from build123d import *

# Parameters (mm, degrees)
ESQUISSE1_R                       = 17
BOSS_EXTRU_1_DEPTH                = 17
ESQUISSE2_R                       = 12.5
BOSS_EXTRU_2_DEPTH                = 11.5
ESQUISSE3_R                       = 12
BOSS_EXTRU_3_DEPTH                = 3.5
ESQUISSE4_R                       = 12.5
BOSS_EXTRU_4_DEPTH                = 1.5
ESQUISSE5_R                       = 10.25
ENL_V_MAT_EXTRU_1_DEPTH           = 30
ESQUISSE6_R                       = 10.25
ESQUISSE6_R_2                     = 6.75
ENL_V_MAT_EXTRU_2_DEPTH           = 1.5
ESQUISSE7_R                       = 12
ESQUISSE7_R_2                     = 10.25
ENL_V_MAT_EXTRU_3_DEPTH           = 2
DIAM_TRE_DU_PER_AGE_3_0_3_1_D     = 3
DIAM_TRE_DU_PER_AGE_3_0_3_1_DEPTH = 12
DIAM_TRE_DU_PER_AGE_3_0_3_1_TIP   = 0.901290929


with BuildPart() as part:
    # Esquisse1 → Boss.-Extru.1 (new body)
    with BuildSketch(Plane.XY):
        Circle(ESQUISSE1_R)
    extrude(amount=BOSS_EXTRU_1_DEPTH)

    # Esquisse2 → Boss.-Extru.2 (add)
    with BuildSketch(Plane.XY.offset(17)):
        Circle(ESQUISSE2_R)
    extrude(amount=BOSS_EXTRU_2_DEPTH)

    # Esquisse3 → Boss.-Extru.3 (add)
    with BuildSketch(Plane.XY.offset(28.5)):
        Circle(ESQUISSE3_R)
    extrude(amount=BOSS_EXTRU_3_DEPTH)

    # Esquisse4 → Boss.-Extru.4 (add)
    with BuildSketch(Plane.XY.offset(32)):
        Circle(ESQUISSE4_R)
    extrude(amount=BOSS_EXTRU_4_DEPTH)

    # Esquisse5 → Enlèv. mat.-Extru.1 (cut)
    with BuildSketch(Plane.XY.offset(33.5)):
        Circle(ESQUISSE5_R)
    extrude(amount=-ENL_V_MAT_EXTRU_1_DEPTH, mode=Mode.SUBTRACT)

    # Esquisse6 → Enlèv. mat.-Extru.2 (cut)
    with BuildSketch(Plane.XY.offset(3.5)):
        Circle(ESQUISSE6_R)
        Circle(ESQUISSE6_R_2, mode=Mode.SUBTRACT)
    extrude(amount=-ENL_V_MAT_EXTRU_2_DEPTH, mode=Mode.SUBTRACT)

    # Esquisse7 → Enlèv. mat.-Extru.3 (cut)
    with BuildSketch(Plane.XY.offset(3.5)):
        Circle(ESQUISSE7_R)
        Circle(ESQUISSE7_R_2, mode=Mode.SUBTRACT)
    extrude(amount=ENL_V_MAT_EXTRU_3_DEPTH, mode=Mode.SUBTRACT)

    # Diamètre du perçage Ø3.0 (3)1
    with Locations(Plane.XY.offset(17)):
        with Locations((0, 14.5)):
            Hole(DIAM_TRE_DU_PER_AGE_3_0_3_1_D / 2, depth=DIAM_TRE_DU_PER_AGE_3_0_3_1_DEPTH)
            with Locations((0, 0, -(DIAM_TRE_DU_PER_AGE_3_0_3_1_DEPTH + DIAM_TRE_DU_PER_AGE_3_0_3_1_TIP / 2))):  # 118° drill point
                Cone(0, DIAM_TRE_DU_PER_AGE_3_0_3_1_D / 2, DIAM_TRE_DU_PER_AGE_3_0_3_1_TIP, mode=Mode.SUBTRACT)


solid = part.part
The model under review builds one solid part; all positions refer to its coordinate system, in mm. A direction names the side the tool comes from. Round coordinates to 2 decimals unless told otherwise and drop trailing zeros. Order: outer loops, then holes, each group sorted by start corner. A loop starts at its lowest first (then second) coordinate and runs counter-clockwise, first axis right, second up. Notation, with made-up numbers: (-10.5, 20.5) -> (25.5, 20.5) arc R11 cw to (25.5, 29.5) -> close; hole circle Ø3 at (2.5, 26.5). An arc over 180 degrees is marked (long way). Write item = value, one per line. Start each with the question number.
Item 1: For line 1 along Y through (x, z) = (0, 11); line 2 along Y through (x, z) = (0, 3); line 3 along Y through (x, z) = (0, 22.5), list the stretches that pass through material, from the lowest coordinate up.
Item 2: Mouldability with a two-part tool opening along Z and no side actions: class faces 4 (the face through (-11.99, 0.53, 30.23)), 5 (the face through (-2.222, -10.006, 19.696)), 6 (the face through (0, 0, 0)) as released by +Z, released by -Z, zero draft, split by the parting line, or undercut.
Item 3: Consider section A-A on z = 8. Write out the cut boundary in (x, y).
Item 4: Clearance check with flat-ended pins moving along their axes: pin 1 Ø12 at (y, z) = (-13.5, 7) entering from +X; pin 2 Ø2 at (y, z) = (4, 12) entering from +X; pin 3 Ø4 at (x, z) = (1, 25.5) entering from +Y. State where each tip first meets the part, or that it passes through.
Item 5: For faces 1 (the face through (0, 13, 11)), 2 (the face through (-7, 10, 32)), 3 (the face through (9.139, 14.334, 8.381)), list the 3-axis set-ups (+Z, -Z, +X, -X, +Y, -Y) from which the entire face can be reached by the end or side of a thin tool; tool diameter is ignored.
Item 6: Consider section D-D on z = 25.5. Write out the cut boundary in (x, y), plus the area to 3 significant figures.
Conclusion:
q1.line_1 = -17 to -10.25, 10.25 to 13, 16 to 17
q1.line_2 = -17 to -10.25, -6.75 to 6.75, 10.25 to 17
q1.line_3 = -12.5 to -10.25, 10.25 to 12.5
q2.face_4 = undercut
q2.face_5 = zero draft
q2.face_6 = released by -Z
q3.outline = circle Ø34 at (0, 0); hole circle Ø20.5 at (0, 0); hole circle Ø3 at (0, 14.5)
q4.pin_1 = 15.26
q4.pin_2 = 16.73
q4.pin_3 = 12.5
q5.face_1 = +Z
q5.face_2 = none
q5.face_3 = +Z, -Z
q6.outline = circle Ø25 at (0, 0); hole circle Ø20.5 at (0, 0)
q6.area = 161 mm2
